```python
from build123d import *

# Parameters (mm, degrees)
SKETCH1_W           = 114.3
SKETCH1_H           = 6.35
BOSS_EXTRUDE1_DEPTH = 50.8
F_1_2_HOLES_DEPTH   = 7.35


with BuildPart() as part:
    # Sketch1 → Boss-Extrude1 (new body, symmetric)
    with BuildSketch(Plane.XY):
        with Locations((0, -3.175)):
            Rectangle(SKETCH1_W, SKETCH1_H)
    extrude(amount=BOSS_EXTRUDE1_DEPTH, both=True)

    # Sketch2 → 1-2 holes (cut, through all)
    with BuildSketch(Plane(origin=(0, 0, 0), x_dir=(1, 0, 0), z_dir=(0, 1, 0))):
        with BuildLine():
            Line((-35.649713965, 34.016189941), (-43.587213965, 29.253689941))
            ThreePointArc((-43.587213965, 29.253689941), (-50.121310059, 30.887213965), (-48.487786035, 37.421310059))
            Line((-48.487786035, 37.421310059), (-40.550286035, 42.183810059))
            ThreePointArc((-40.550286035, 42.183810059), (-34.016189941, 40.550286035), (-35.649713965, 34.016189941))
        make_face()
        with BuildLine():
            Line((-35.649713965, -34.016189941), (-43.587213965, -29.253689941))
            ThreePointArc((-43.587213965, -29.253689941), (-50.121310059, -30.887213965), (-48.487786035, -37.421310059))
            Line((-48.487786035, -37.421310059), (-40.550286035, -42.183810059))
            ThreePointArc((-40.550286035, -42.183810059), (-34.016189941, -40.550286035), (-35.649713965, -34.016189941))
        make_face()
        with BuildLine():
            Line((35.649713965, 34.016189941), (43.587213965, 29.253689941))
            ThreePointArc((43.587213965, 29.253689941), (50.121310059, 30.887213965), (48.487786035, 37.421310059))
            Line((48.487786035, 37.421310059), (40.550286035, 42.183810059))
            ThreePointArc((40.550286035, 42.183810059), (34.016189941, 40.550286035), (35.649713965, 34.016189941))
        make_face()
        with BuildLine():
            Line((35.649713965, -34.016189941), (43.587213965, -29.253689941))
            ThreePointArc((43.587213965, -29.253689941), (50.121310059, -30.887213965), (48.487786035, -37.421310059))
            Line((48.487786035, -37.421310059), (40.550286035, -42.183810059))
            ThreePointArc((40.550286035, -42.183810059), (34.016189941, -40.550286035), (35.649713965, -34.016189941))
        make_face()
    extrude(amount=-F_1_2_HOLES_DEPTH, mode=Mode.SUBTRACT)


solid = part.part
```
Check sheet for the modelled part. Datum: model origin and axes. Units: mm. A direction names the side the tool comes from. Give positions to 0.01 mm unless a question says otherwise; leave off trailing zeros. Loops run counter-clockwise (first coordinate to the right, second up) from the corner with the lowest first, then second, coordinate; pieces in that order, holes last. Notation, with made-up numbers: (-28.75, 0) - (-11.75, 0) arc R26 ccw to (-11.75, 37) - close; hole circle Ø6 at (35.25, 61). An arc over 180 degrees is marked (long way). One line per question, with ' | ' between items. Start each with the question number.
1. Material ranges on line 1 along Z through (x, y) = (-45.5, -2.5); line 2 along X through (y, z) = (-0.5, -37.5); line 3 along X through (y, z) = (-3, -35.5), recorded low to high. Write a range as [from, to].
2. Cross-section at B-B, the plane x = -38.1. Enter the section's corners in (y, z), plus the area to 3 significant figures.
3. Draft check along Z on faces 1 (the cylindrical face through (-34.07, -3.13, -40.64)), 2 (the flat face through (-57.15, -3, 1)), 3 (the flat face through (-1, -3, -50.8)). Enter one of: released by +Z, released by -Z, zero draft, split by the parting line, or undercut.
4. Set-up check for faces 4 (the flat face through (-39.56, -3.13, -31.67)), 5 (the flat face through (-1, -3, 50.8)): record each of +Z, -Z, +X, -X, +Y, -Y from which the full face is reachable in a straight line by a thin tool's end or side.
5. Cross-section at A-A, the plane y = -1.25. Give the number of separate pieces and of enclosed holes in the cut face, plus the area to 3 significant figures.
Check result:
1) line 1: z = [-50.8, -39.21], [-28.61, 28.61], [39.21, 50.8] | line 2: x = [-57.15, -48.36], [-33.38, 33.38], [48.36, 57.15] | line 3: x = [-57.15, -50.28], [-34.11, 34.11], [50.28, 57.15]
2) outline: (-6.35, -50.8) - (0, -50.8) - (0, -42.86) - (-6.35, -42.86) - close; (-6.35, -32.55) - (0, -32.55) - (0, 32.55) - (-6.35, 32.55) - close; (-6.35, 42.86) - (0, 42.86) - (0, 50.8) - (-6.35, 50.8) - close | area: 514 mm2
3) face 1: undercut | face 2: zero draft | face 3: released by -Z
4) face 4: +Y, -Y | face 5: +Z, +X, -X, +Y, -Y
5) separate pieces: 1 | enclosed holes: 4 | area: 11,000 mm2
